Design review of the part built by this model. Coordinates are the model's own, in mm. Coordinates: 2 decimals unless noted, no trailing zeros. Order: outer loops, then holes, each group sorted by start corner. A loop starts at its lowest first (then second) coordinate and runs counter-clockwise, first axis right, second up. Notation, with made-up numbers: (72.25, 77) - (80.25, 77) arc R14 cw to (80.25, 104) - close; hole circle Ø5 at (6.25, 16.25). An arc over 180 degrees is marked (long way). Write each question's results on one line, items separated by ' | '. Start each with the question number.
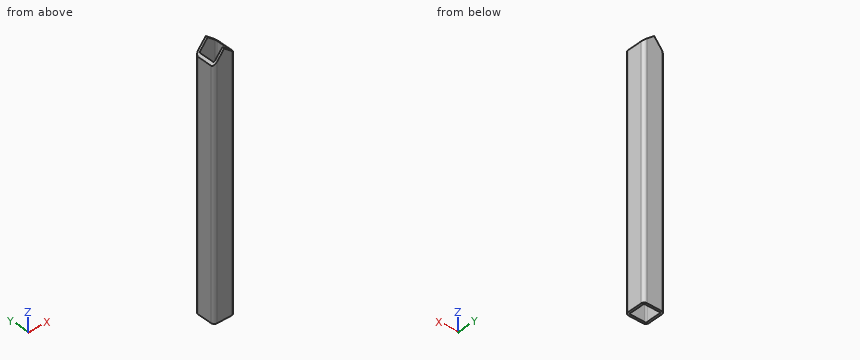
Autodesk Inventor part; units mm, degrees
ref_plane "Start Plane" through (0, 0, 0) normal (0, 0, 1) x (1, 0, 0)
ref_plane "End Plane" through (0, 0, 245.204) normal (0, 0, 1) x (1, 0, 0)
ref_plane "Work Plane4" through (10, 0, 257.4621) normal (-0.7749, 0, 0.6321) x (0.6321, 0, 0.7749)
ref_plane "Start Plane" through (0, 0, 0) normal (0, 0, 1) x (1, 0, 0)
ref_plane "End Plane" through (0, 0, 245.204) normal (0, 0, 1) x (1, 0, 0)
sketch "Sketch" plane through (0, 0, 0) normal (0, 0, 1) x (1, 0, 0)
  line L0 (-10, -7) -> (-10, 7)
  line L1 (-7, 10) -> (7, 10)
  line L2 (10, 7) -> (10, -7)
  line L3 (7, -10) -> (-7, -10)
  arc A0 (-10, -7) -> (-7, -10) centre (-7, -7) ccw
  arc A1 (-7, 10) -> (-10, 7) centre (-7, 7) ccw
  arc A2 (10, 7) -> (7, 10) centre (7, 7) ccw
  arc A3 (7, -10) -> (10, -7) centre (7, -7) ccw
  arc A4 (-7, 8) -> (-8, 7) centre (-7, 7) ccw
  line L4 (-7, 8) -> (7, 8)
  arc A5 (8, 7) -> (7, 8) centre (7, 7) ccw
  line L5 (8, 7) -> (8, -7)
  arc A6 (7, -8) -> (8, -7) centre (7, -7) ccw
  line L6 (7, -8) -> (-7, -8)
  arc A7 (-8, -7) -> (-7, -8) centre (-7, -7) ccw
  line L7 (-8, -7) -> (-8, 7)
  line L8 (0, 14.8698) -> (0, -14.8698) construction
  line L9 (-14.8698, 0) -> (14.8698, 0) construction
  dimension "d7" = 3
  dimension "d10" = 20
  dimension "d11" = 20
  dimension "d12" = 2
  dimension "d15" = 10
  dimension "d16" = 10
extrude "Body" add sketch "Sketch" along normal up to surface (245.204 mm away) from surface at 0
sketch "Sketch3" plane through (0, 0, 0) normal (0, 0, 1) x (1, 0, 0)
  line L0 (0, 0) -> (10, 0)
ref_plane "Work Plane3" through (0, 0, 0) normal (0, -1, 0) x (1, 0, 0)
sketch "Sketch4" plane through (0, 0, 0) normal (0, -1, 0) x (1, 0, 0)
  line L0 (-2, 0) -> (12, 0)
  line L1 (-2, 245.204) -> (12, 245.204)
  dimension "d18" = 245.204
ref_plane "Work Plane4" through (10, 0, 257.4621) normal (-0.7749, 0, 0.6321) x (0.6321, 0, 0.7749)
split "Split1" plane through (10, 0, 257.4621) removes the side toward (-0.7749, 0, 0.6321)
ref_plane "Work Plane5" through (-10, 0, 253.3619) normal (0.6321, 0, 0.7749) x (0.7749, 0, -0.6321)
split "Split2" plane through (-10, 0, 253.3619) removes the side toward (0.6321, 0, 0.7749)
equation "\"d7\" = G_IR"
equation "\"d10\" = G_H"
equation "\"d11\" = G_W"
equation "\"d12\" = G_T"
equation "\"d15\" = 0.5 * d10"
equation "\"d16\" = 0.5 * d11"
equation "\"d3\" = G_L"
equation "\"G_W\" = 20"
equation "\"G_H\" = 20"
equation "\"G_T\" = 2"
equation "\"G_IR\" = 3"
equation "\"G_L\" = d18"
equation "\"G_OFFSET_START\" = 0"
equation "\"G_OFFSET_END\" = 0"
equation "\"d14\" = G_OFFSET_END + B_L"
equation "\"B_L\" = 245.204"
properties part number "ISO 12633-2 - 20x20x2 - 245.2" material "Steel, Mild"
(1) Clearance check with flat-ended pins moving along their axes: pin 1 (5 mm diameter, centred on x = 5, y = -2, fed in from -Z); pin 2 (8 mm diameter, centred on x = 4.5, y = 6, fed in from +Z). State where each tip first meets the part, or that it passes through.
(2) Take a section at A-A (z = 186). State the section outline as (x, y) points, plus the area to 3 significant figures.
(3) To check wall thickness, follow line 1 along Y through (x, z) = (-4, 223.5); line 2 along Z through (x, y) = (8, -8). State the ranges of each line that lie inside material, in increasing order. Write a range as [from, to].
(4) Take a section at B-B (y = 4.75). State the section outline as (x, z) points.
(5) Take a section at C-C (x = -2.25). State the section outline as (y, z) points, plus the area to 3 significant figures.
Worked out:
1) pin 1: through | pin 2: z = 244.36
2) outline: (-10, -7) arc R3 ccw to (-7, -10) - (7, -10) arc R3 ccw to (10, -7) - (10, 7) arc R3 ccw to (7, 10) - (-7, 10) arc R3 ccw to (-10, 7) - close; hole (-8, -7) arc R1 ccw to (-7, -8) - (7, -8) arc R1 ccw to (8, -7) - (8, 7) arc R1 ccw to (7, 8) - (-7, 8) arc R1 ccw to (-8, 7) - close | area: 137 mm^2
3) line 1: [-10, -8], [8, 10] | line 2: [0, 238.68]
4) outline: (-10, 0) - (-8, 0) - (-8, 235.4) - (-10, 232.94) - close; (8, 0) - (10, 0) - (10, 237.05) - (8, 238.68) - close
5) outline: (-10, 0) - (-8, 0) - (-8, 242.44) - (-10, 242.44) - close; (8, 0) - (10, 0) - (10, 242.44) - (8, 242.44) - close | area: 970 mm^2
